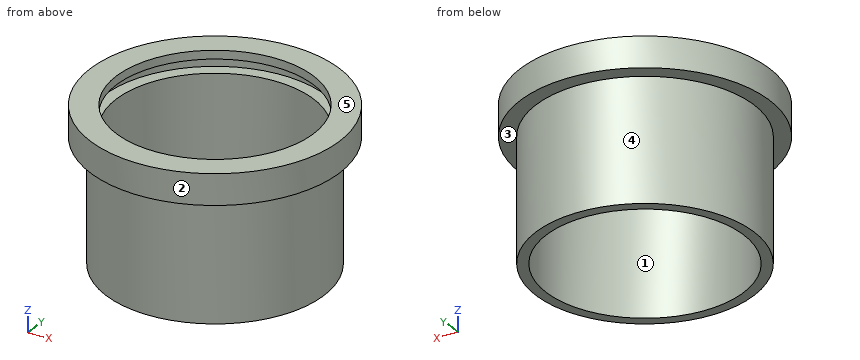
from build123d import *

# Parameters (mm, degrees)
F0_R          = 16.048100164
F0_R_2        = 14.5297232328
F1_DEPTH      = 20
F2_START      = 18
F0_R_3        = 18.3403382945
F2_DEPTH      = 4.5
F3_SCALE      = 0.5
F5_R          = 8.1793967512
F6_DEPTH      = 0.5
F6_DEPTH_BACK = 0.5


with BuildPart() as f1:
    # F0 (on Top) → F1 (new body)
    with BuildSketch(Plane.XY):
        Circle(F0_R)
        Circle(F0_R_2, mode=Mode.SUBTRACT)
    extrude(amount=F1_DEPTH)

    # F0 (on Top) → F2 (join)
    with BuildSketch(Plane.XY.offset(F2_START)):
        Circle(F0_R_3)
        Circle(F0_R, mode=Mode.SUBTRACT)
        Circle(F0_R)
        Circle(F0_R_2, mode=Mode.SUBTRACT)
    extrude(amount=F2_DEPTH)


with BuildPart() as f1_1:
    # F3: moved
    add(f1.part.scale(F3_SCALE))

    # F5 (on offset) → F6 (cut, two sides)
    with BuildSketch(Plane.XY.offset(10.125)) as f6_sk:
        Circle(F5_R)
    extrude(amount=F6_DEPTH, mode=Mode.SUBTRACT)
    extrude(f6_sk.sketch, amount=-F6_DEPTH_BACK, mode=Mode.SUBTRACT)


solid = f1_1.part
Part model, mm, in its own coordinate system. Face numbers are marked on the shaded views. A direction names the side the tool comes from. Coordinates: 2 decimals unless noted, no trailing zeros. Order: outer loops, then holes, each group sorted by start corner. A loop starts at its lowest first (then second) coordinate and runs counter-clockwise, first axis right, second up. Notation, with made-up numbers: M 63.25,-30 L 98.25,-30 A28 cw 98.25,-11 Z; hole C 89.25,55.5 d3. An arc over 180 degrees is marked long. One line per question, with ' | ' between items.
Q1. Slice it at C-C (z = 3). Give the cut face in (x, y), and give its area (3 significant figures).
A:
outline: C 0,0 d16.05; hole C 0,0 d14.53 | area: 36.5 mm^2
Q2. 3-axis set-ups, long thin cutter, end or side, ignore diameter. For the marked faces 4 and 5: which of +Z, -Z, +X, -X, +Y, -Y reach the whole face in a straight line?
A:
face 4: -Z | face 5: +Z, +X, -X, +Y, -Y
Q3. Two-plate mould, pull along X, no slides. Class the marked faces 1, 2 and 3: +X half, -X half, draft (parallel to the pull), parting line (faces both ways), or undercut.
A:
face 1: undercut | face 2: parting line | face 3: draft
Q4. Pin check, flat tips, straight feed: P1, Ø4, axis at x = -4.5, z = 8, coming from the +Y side; P2, Ø6, axis at x = -3.5, z = 2.5, coming from the +Y side; P3, Ø6, axis at x = -5, z = 2.5, coming from the +Y side. Stop position of each tip, or through.
A:
P1: stops at y = 8.74 | P2: stops at y = 8.01 | P3: stops at y = 7.77
Q5. Drill centre lines: line 1 (X direction, y = 0, z = 6.25); line 2 (Y direction, x = 0, z = 10.8); line 3 (Z direction, x = 0.25, y = -7.5) (3 decimals). Where is each one in solid material? Low to high.
A:
line 1: x = -8.02 to -7.26, 7.26 to 8.02 | line 2: y = -9.17 to -7.26, 7.26 to 9.17 | line 3: z = 0 to 9.625, 10.625 to 11.25
Q6. Slice it at A-A (y = 0). Give the cut face in (x, z) (3 decimals), and give its area (3 significant figures).
A:
outline: M -9.17,9 L -8.024,9 L -8.024,0 L -7.265,0 L -7.265,9.625 L -8.179,9.625 L -8.179,10.625 L -7.265,10.625 L -7.265,11.25 L -9.17,11.25 Z; M 7.265,0 L 8.024,0 L 8.024,9 L 9.17,9 L 9.17,11.25 L 7.265,11.25 L 7.265,10.625 L 8.179,10.625 L 8.179,9.625 L 7.265,9.625 Z | area: 20.4 mm^2
Q7. Slice it at B-B (x = 7). Give the cut face in (y, z) (3 decimals).
A:
outline: M -5.924,9 L -3.922,9 L -3.922,0 L -1.944,0 L -1.944,9.625 L -4.231,9.625 L -4.231,10.625 L -1.944,10.625 L -1.944,11.25 L -5.924,11.25 Z; M 1.944,0 L 3.922,0 L 3.922,9 L 5.924,9 L 5.924,11.25 L 1.944,11.25 L 1.944,10.625 L 4.231,10.625 L 4.231,9.625 L 1.944,9.625 Z
